```python
from build123d import *

# Parameters (mm, degrees)
SKETCH1_R         = 9.525
EXTRUDE1_DEPTH    = 19.05
CHAMFER1_SIZE     = 0.4064
SKETCH6_R         = 1.984375
BLIND_HOLES_DEPTH = 12.7


with BuildPart() as part:
    # Sketch1 → Extrude1 (new body, symmetric)
    with BuildSketch(Plane.XY):
        Circle(SKETCH1_R)
    extrude(amount=EXTRUDE1_DEPTH, both=True)

    # Chamfer1
    chamfer1_edges = [part.edges().sort_by_distance(p)[0] for p in [
        (-9.525, 0, -19.05),
        (-9.525, 0, 19.05),
    ]]
    chamfer(chamfer1_edges, length=CHAMFER1_SIZE)

    # Sketch6 → Blind Holes (cut)
    with BuildSketch(Plane(origin=(0, -9.525, 0), x_dir=(-1, 0, 0), z_dir=(0, 1, 0))):
        with Locations(Location((0, 12.7, 0), (0, 0, 270))):  # turned: the seam where the file's is
            Circle(SKETCH6_R)
        with Locations(Location((0, -12.7, 0), (0, 0, 270))):  # turned: the seam where the file's is
            Circle(SKETCH6_R)
    extrude(amount=BLIND_HOLES_DEPTH, mode=Mode.SUBTRACT)


solid = part.part
```
Geometry: final body of the model. Coordinates: model frame, mm. A direction names the side the tool comes from. Give positions to 0.01 mm unless a question says otherwise; leave off trailing zeros. Loops run counter-clockwise (first coordinate to the right, second up) from the corner with the lowest first, then second, coordinate; pieces in that order, holes last. Notation, with made-up numbers: (7.25, 69.5) - (62.25, 69.5) arc R16 cw to (62.25, 93.5) - close; hole circle Ø11 at (-8.5, 44.5). An arc over 180 degrees is marked (long way). Answer as CSV lines item,"result". Start each with the question number.
(1) Section query D-D (y = 2.75). Give the number of separate pieces and of enclosed holes in the cut face, and give its area (3 significant figures).
(2) Ray query, line 1 along Z through (x, y) = (-1.25, -6); line 2 along X through (y, z) = (-7, -12.7); line 3 along X through (y, z) = (-1, -14). Return the intervals inside material, ascending. Write a range as [from, to].
(3) Mould query, pull axis X, two halves, no side actions, for faces 1 (the face through (-7.559, -5.796, 0.261)), 2 (the face through (0, 3.175, -13)), 3 (the face through (0, 0, -19.05)). Classes: +X half, -X half, draft (parallel to the pull), parting line (faces both ways), or undercut.
(4) Pin query (flat end, axial travel): P1, Ø3, axis at x = -0.5, z = -13, coming from the -Y side; P2, Ø10, axis at y = -6.5, z = 0, coming from the -X side; P3, Ø8, axis at y = 6, z = 0.5, coming from the +X side. Return the tip coordinate at first contact, or that it passes through.
(5) Section query A-A (y = 0). Output: boundary loops of the cut face in (x, z) (3 decimals), and give its area (3 significant figures).
(6) Reachability of faces 4 (the face through (0, 0, 19.05)), 5 (the face through (-0.087, -3.264, -10.718)) from +Z, -Z, +X, -X, +Y, -Y: full face, straight path, thin tool, end or side. Return the list, or none.
(7) Section query C-C (z = -3.5). Output: boundary loops of the cut face in (x, y) (3 decimals), and give its area (3 significant figures).
(8) Section query B-B (x = 0). Output: boundary loops of the cut face in (y, z) (3 decimals).
Worked answers:
1,separate pieces,"1"
1,enclosed holes,"2"
1,area,"670 mm^2"
2,line 1,"z = [-19.05, -14.24], [-11.16, 11.16], [14.24, 19.05]"
2,line 2,"x = [-6.46, -1.98], [1.98, 6.46]"
2,line 3,"x = [-9.47, -1.5], [1.5, 9.47]"
3,face 1,"parting line"
3,face 2,"undercut"
3,face 3,"draft"
4,P1,"stops at y = -9.47"
4,P2,"stops at x = -9.41"
4,P3,"stops at x = 9.31"
5,outline,"(-9.525, -18.644) - (-9.119, -19.05) - (9.119, -19.05) - (9.525, -18.644) - (9.525, 18.644) - (9.119, 19.05) - (-9.119, 19.05) - (-9.525, 18.644) - close; hole circle Ø3.969 at (0, -12.7); hole circle Ø3.969 at (0, 12.7)"
5,area,"701 mm^2"
6,face 4,"+Z, +X, -X, +Y, -Y"
6,face 5,"-Y"
7,outline,"circle Ø19.05 at (0, 0)"
7,area,"285 mm^2"
8,outline,"(-9.525, -18.644) - (-9.119, -19.05) - (9.119, -19.05) - (9.525, -18.644) - (9.525, 18.644) - (9.119, 19.05) - (-9.119, 19.05) - (-9.525, 18.644) - (-9.525, 14.684) - (3.175, 14.684) - (3.175, 10.716) - (-9.525, 10.716) - (-9.525, -10.716) - (3.175, -10.716) - (3.175, -14.684) - (-9.525, -14.684) - close"
